Build history of the part. All positions in model axes, mm. Coordinates: 2 decimals unless noted, no trailing zeros. Loops run counter-clockwise (first coordinate to the right, second up) from the corner with the lowest first, then second, coordinate; pieces in that order, holes last.
(1) Two-plate mould, pull along Y, no slides. Class faces 1 (the face through (0.076, 0.009, 3.632)), 2 (the face through (1.878, 1.438, -0.748)), 3 (the face through (3.724, 3.15, -1.808)): pulls with the +Y half, pulls with the -Y half, needs draft (parallel to the pull), parting line crosses it, or undercut.
(2) Slice it at A-A (x = 0.6). Give the cut face in (y, z).
(3) Flat gauge pin, fed straight in: P1, Ø1.5, axis at x = 2, y = -2, coming from the -Z side. Where does the tip first touch, or does it go through?
(4) Wall check: L1, parallel to Z at x = 2.35, y = 0.75; L2, parallel to Y at x = 2.8, z = 0; L3, parallel to Z at x = 1.2, y = -0.5. Give the ranges that are in metal, low to high.
Autodesk Inventor part; units mm, degrees
ref_plane "MSC_PT1" through (3.8, 0, 0) normal (1, 0, 0) x (0, 1, 0)
ref_plane "MSC_PT2" through (0, 0, 0) normal (-1, 0, 0) x (0, -1, 0)
ref_plane "MSC_PF1" through (0, 0, 0) normal (1, 0, 0) x (0, 1, 0)
sketch "Boceto1" plane through (0, 0, 0) normal (1, 0, 0) x (0, 1, 0)
  line L0 (3.5, 2.0207) -> (3.5, -2.0207)
  line L1 (3.5, -2.0207) -> (0, -4.0415)
  line L2 (0, -4.0415) -> (-3.5, -2.0207)
  line L3 (-3.5, -2.0207) -> (-3.5, 2.0207)
  line L4 (-3.5, 2.0207) -> (0, 4.0415)
  line L5 (0, 4.0415) -> (3.5, 2.0207)
  circle A0 centre (0, 0) radius 3.5 construction
  dimension "d0" = 7
extrude "Extrusión1" add sketch "Boceto1" along normal blind 3.8
sketch "Boceto2" plane through (3.8, 0, 0) normal (1, 0, 0) x (0, 1, 0)
  line L0 (-3.5, 2.0207) -> (0, 4.0415)
  line L1 (0, -4.0415) -> (-3.5, -2.0207)
  line L2 (-3.5, 2.0207) -> (3.5, -2.0207) construction
  line L3 (-3.5, -2.0207) -> (3.5, 2.0207) construction
  point P0 (0, 0)
hole "Agujero1" at (3.8, 0, 0) direction (-1, 0, 0) diameter 3.242 end through all
chamfer "Chaflán1" distance 0.35 angle 45 2 edges at (3.8, 0, 1.621) (0, 0, 1.621)
sketch "Boceto3" plane through (0, 0, 0) normal (0, 1, 0) x (-1, 0, 0)
  line L0 (-7.0172, 0) -> (2.1698, 0)
  line L1 (-5.7048, 0) -> (0.8574, 0)
  line L2 (-3.8, 0) -> (-3.8, -4.0415)
  line L3 (-3.8, -4.0415) -> (0, -4.0415)
  line L4 (0, -4.0415) -> (0, 0)
  line L5 (-3.8, -2.0207) -> (-3.8, -4.0415)
  line L6 (0, -2.0207) -> (0, -4.0415)
  line L7 (0, -4.0415) -> (-3.8, -4.0415)
  line L8 (-3.8, -3.5) -> (-3.4874, -4.0415)
  line L9 (-3.8, -4.0415) -> (-3.8, -3.5)
  line L10 (-3.8, -4.0415) -> (-3.4874, -4.0415)
  line L11 (0, -3.5) -> (-0.3126, -4.0415)
  line L12 (-0.3126, -4.0415) -> (0, -4.0415)
  line L13 (0, -4.0415) -> (0, -3.5)
  dimension "d32" = 3.5
  dimension "d33" = 30
revolve "Revolución1" cut sketch "Boceto3" angle 360 about axis through (0, 0, 0) along (-1, 0, 0) contours L8 L3 L2 | L4 L3 L11
ref_plane "MSC_PT1" through (3.8, 0, 0) normal (1, 0, 0) x (0, 1, 0)
ref_plane "MSC_PT2" through (0, 0, 0) normal (-1, 0, 0) x (0, -1, 0)
ref_plane "MSC_PF1" through (0, 0, 0) normal (1, 0, 0) x (0, 1, 0)
equation "\"d0\" = Smax"
equation "\"d1\" = Mmax"
equation "\"d10\" = 0.5 * PTC"
equation "\"d32\" = 0.5 * Smax"
equation "\"NND\" = 4"
equation "\"Smax\" = 7"
equation "\"Mmax\" = 3.8"
equation "\"PTC\" = 0.7"
equation "\"THREADDIA\" = NND"
equation "\"TEMPLATE\" = 1.2345"
properties part number "ANSI B18.2.4.2M - M4x0,7" material "Acero, suave"
Response values:
1. face 1: parting line crosses it
1. face 2: undercut
1. face 3: pulls with the +Y half
2. outline: (-3.5, -2.02) - (0, -4.04) - (3.5, -2.02) - (3.5, 2.02) - (0, 4.04) - (-3.5, 2.02) - close; hole circle Ø3.24 at (0, 0)
3. P1: stops at z = -3.32
4. L1: z = -3.61 to -1.44, 1.44 to 3.61
4. L2: y = -3.5 to -1.62, 1.62 to 3.5
4. L3: z = -3.75 to -1.54, 1.54 to 3.75
